Could you check a few things on this model? Use its own coordinates, in mm. Round coordinates to 2 decimals unless told otherwise and drop trailing zeros. Order: outer loops, then holes, each group sorted by start corner. A loop starts at its lowest first (then second) coordinate and runs counter-clockwise, first axis right, second up.
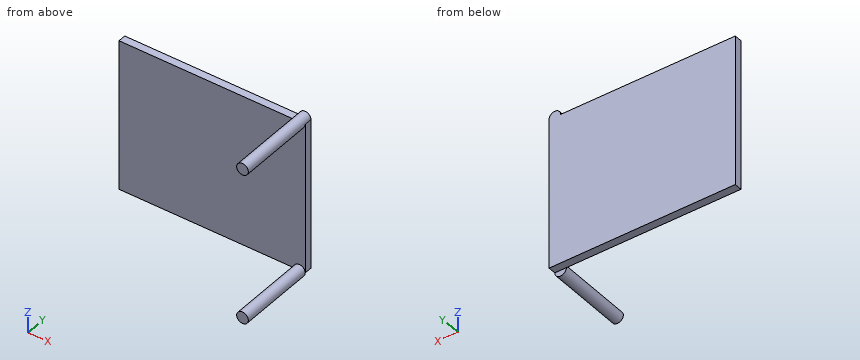
Autodesk Inventor part; units mm, degrees
ref_plane "YZ Plane" through (0, 0, 0) normal (1, 0, 0) x (0, 1, 0)
ref_plane "XZ Plane" through (0, 0, 0) normal (0, 1, 0) x (-1, 0, 0)
ref_plane "XY Plane" through (0, 0, 0) normal (0, 0, 1) x (1, 0, 0)
sketch "草圖1" plane through (0, 0, 0) normal (0, 1, 0) x (-1, 0, 0)
  circle A0 centre (0.913, -0.7631) radius 0.75
  point P0 (0, 0)
  dimension "d0" = 1.5
extrude "擠出1" add sketch "草圖1" along normal blind 10
sketch "草圖2" plane through (-0.913, 10, -0.7631) normal (0, 1, 0) x (1, 0, 0)
  circle A0 centre (0, 0) radius 0.75
  line L0 (-0.75, 0) -> (0.75, 0)
  line L1 (0.75, 0) -> (0.75, 19.5)
  line L2 (0.75, 19.5) -> (-0.75, 19.5)
  line L3 (-0.75, 19.5) -> (-0.75, 0)
  circle A1 centre (0, 0) radius 0.75
  point P0 (0.913, -0.7631)
  dimension "d3" = 19.5
extrude "擠出2" add sketch "草圖2" along normal blind 1
pattern_linear "矩形陣列1" count 2 spacing 19.5 along (0, 0, -1) of "擠出1"
sketch "草圖3" plane through (-0.913, 11, -0.7631) normal (0, 1, 0) x (1, 0, 0)
  circle A0 centre (0, 19.5) radius 0.75
  line L0 (-0.75, 19.5) -> (-23.25, 19.5)
  line L1 (-23.25, 19.5) -> (-23.25, 0)
  line L2 (-23.25, 0) -> (-0.75, 0)
  line L3 (-0.75, 0) -> (-0.75, 19.5)
  line L4 (0.75, 0) -> (0.75, 19.5)
  point P0 (0.913, -0.7631)
  point P1 (-0.75, 0)
  dimension "d9" = 24
extrude "擠出3" add sketch "草圖3" against normal up to surface (1 mm away) contours L3 L2 L1 L0
Q1. Imagine slicing it at B-B, the plane z = -13.25. Please give me the cut outline in (x, y).
Q2. For P1, Ø8, axis at x = -5, z = -4, coming from the -Y side; P2, Ø6, axis at x = -20, y = 9.5, coming from the +Z side; P3, Ø0.5, axis at x = -14, y = 10.5, coming from the -Z side, each with a flat end and sliding along its axis, tell me the tip position at first contact or that it passes through.
Q3. Imagine slicing it at A-A, the plane y = 4. Please give me the cut outline in (x, z), then the cut area to 3 significant figures.
Q4. I need wall thicknesses on L1, parallel to Y at x = -21.25, z = -8.75; L2, parallel to X at y = 0.75, z = -0.75; L3, parallel to Z at x = -13.75, y = 10.25. Which ranges of each line are inside material? Lowest first, please.
Q5. Imagine slicing it at C-C, the plane x = -16.5. Please give me the cut outline in (y, z).
Filled in:
1. outline: (-24.16, 10) - (-0.16, 10) - (-0.16, 11) - (-24.16, 11) - close
2. P1: stops at y = 10
2. P2: stops at z = -0.76
2. P3: stops at z = -20.26
3. outline: circle Ø1.5 at (-0.91, -20.26); circle Ø1.5 at (-0.91, -0.76)
3. area: 3.53 mm2
4. L1: y = 10 to 11
4. L2: x = -1.66 to -0.16
4. L3: z = -20.26 to -0.76
5. outline: (10, -20.26) - (11, -20.26) - (11, -0.76) - (10, -0.76) - close
